from build123d import *

# Parameters (mm, degrees)
F0_R     = 147.5
F1_DEPTH = 35
F2_R     = 50
F3_DEPTH = 56
F4_R     = 45
F5_DEPTH = 40
F7_DEPTH = 40


with BuildPart() as f1:
    # F0 (on Front) → F1 (new body)
    with BuildSketch(Plane.XZ):
        Circle(F0_R)
    extrude(amount=F1_DEPTH)

    # F2 (on face) → F3 (join)
    with BuildSketch(Plane(origin=(0, 0, 0), x_dir=(-1, 0, 0), z_dir=(0, 1, 0))):
        Circle(F2_R)
    extrude(amount=F3_DEPTH)

    # F4 (on face) → F5 (join)
    with BuildSketch(Plane(origin=(0, 56, 0), x_dir=(-1, 0, 0), z_dir=(0, 1, 0))):
        Circle(F4_R)
    extrude(amount=F5_DEPTH)

    # F6 (on face) → F7 (cut)
    with BuildSketch(Plane.XZ.offset(35)):
        with BuildLine():
            ThreePointArc((36.4554849148, -71.2109375), (0, -80), (-36.4554849148, -71.2109375))
            ThreePointArc((-36.4554849148, -71.2109375), (-4.4254556656, -117.2379556656), (37.5, -80))
            ThreePointArc((37.5, -80), (37.2379556656, -75.5745443344), (36.4554849148, -71.2109375))
        make_face()
        with BuildLine():
            ThreePointArc((36.4554849148, -71.2109375), (0, -42.5), (-36.4554849148, -71.2109375))
            ThreePointArc((-36.4554849148, -71.2109375), (0, -80), (36.4554849148, -71.2109375))
        make_face()
    extrude(amount=-F7_DEPTH, mode=Mode.SUBTRACT)


solid = f1.part
Geometry check sheet. Reference: the model listing, model coordinates, mm. A direction names the side the tool comes from. Coordinates: 2 decimals unless noted, no trailing zeros. Order: outer loops, then holes, each group sorted by start corner. A loop starts at its lowest first (then second) coordinate and runs counter-clockwise, first axis right, second up. Notation, with made-up numbers: (61, 43.25) -> (77, 43.25) arc R20 ccw to (77, 56.25) -> close; hole circle Ø5 at (-18.5, 40). An arc over 180 degrees is marked (long way). Use a Markdown table: item, result. Add a question column.
1. Go/stop test with flat-tipped pins: pin 1 Ø5 at (x, z) = (30, -59.5) entering from -Y; pin 2 Ø3 at (y, z) = (18, 29) entering from +X; pin 3 Ø6 at (y, z) = (71.5, 19.5) entering from +X; pin 4 Ø12 at (y, z) = (73, 46) entering from -X. Record where each tip stops, or that it passes through.
2. Cross-section at B-B (z = 0). Enter the section's corners in (x, y), and give its area (3 significant figures).
3. Material ranges on L1, parallel to Z at x = 0, y = -4; L2, parallel to Y at x = 72.5, z = 60.5; L3, parallel to X at y = -18, z = -80, recorded low to high.
4. Cross-section at C-C (z = -62.5). Enter the section's corners in (x, y).
5. Cross-section at D-D (y = -16.5). Enter the section's corners in (x, z), and give its area (3 significant figures).
6. Cross-section at A-A (x = 0). Enter the section's corners in (y, z).
7. Set-up check for faces 1 (the face through (1, 96, 1)), 2 (the face through (41, 56, 19)), 3 (the face through (0, 5, -46)): record each of +Z, -Z, +X, -X, +Y, -Y from which the full face is reachable in a straight line by a thin tool's end or side.
Filled sheet:
| question | item | result |
|---|---|---|
| 1 | pin 1 | y = -35 |
| 1 | pin 2 | x = 41.76 |
| 1 | pin 3 | x = 41.87 |
| 1 | pin 4 | x = -20.62 |
| 2 | outline | (-147.5, -35) -> (147.5, -35) -> (147.5, 0) -> (50, 0) -> (50, 56) -> (45, 56) -> (45, 96) -> (-45, 96) -> (-45, 56) -> (-50, 56) -> (-50, 0) -> (-147.5, 0) -> close |
| 2 | area | 19,500 mm2 |
| 3 | L1 | -147.5 to -117.5, -42.5 to 147.5 |
| 3 | L2 | -35 to 0 |
| 3 | L3 | -123.92 to -37.5, 37.5 to 123.92 |
| 4 | outline | (-133.6, -35) -> (-33.17, -35) -> (-33.17, 0) -> (-133.6, 0) -> close; (33.17, -35) -> (133.6, -35) -> (133.6, 0) -> (33.17, 0) -> close |
| 5 | outline | circle Ø295 at (0, 0); hole circle Ø75 at (0, -80) |
| 5 | area | 63,900 mm2 |
| 6 | outline | (-35, -147.5) -> (0, -147.5) -> (0, -117.5) -> (-35, -117.5) -> close; (-35, -42.5) -> (5, -42.5) -> (5, -50) -> (56, -50) -> (56, -45) -> (96, -45) -> (96, 45) -> (56, 45) -> (56, 50) -> (0, 50) -> (0, 147.5) -> (-35, 147.5) -> close |
| 7 | face 1 | +Z, -Z, +X, -X, +Y |
| 7 | face 2 | +Y |
| 7 | face 3 | -Z, -Y |
